Input: part model. Units: mm. Frame: model coordinates. Face numbers are marked on the shaded views. A direction names the side the tool comes from. Round coordinates to 2 decimals unless told otherwise and drop trailing zeros. Order: outer loops, then holes, each group sorted by start corner. A loop starts at its lowest first (then second) coordinate and runs counter-clockwise, first axis right, second up. Notation, with made-up numbers: (49, 88) -> (88, 88) arc R28 ccw to (88, 112) -> close; hole circle Ø3 at (-39, -21). An arc over 180 degrees is marked (long way). Use a Markdown table: item, result.
from build123d import *

# Parameters (mm, degrees)
F1_DEPTH      = 70
F3_DEPTH      = 40
F4_SIZE       = 1
F6_DEPTH      = 25
F6_DEPTH_BACK = 100
F7_R          = 4
F8_DEPTH      = 30
F8_DEPTH_BACK = 25
F10_R         = 5
F11_DEPTH     = 30
F11_TAPER     = 1
F13_START     = 25
F12_R         = 21.0146982342
F13_DEPTH     = 15


with BuildPart() as f1:
    # F0 (on Top) → F1 (new body)
    with BuildSketch(Plane.XY):
        Polygon((0, -15), (0, 0), (0, 15), (-10, 9.2264973081), (-10, -9.2264973081), align=None)
    extrude(amount=F1_DEPTH)

    # F2 (on Right) → F3 (join)
    with BuildSketch(Plane.YZ):
        with BuildLine():
            ThreePointArc((7, 35), (-4.9497474683, 39.9497474683), (0, 28))
            ThreePointArc((0, 28), (4.9497474683, 30.0502525317), (7, 35))
        make_face()
        with BuildLine():
            ThreePointArc((4, 35), (2.8284271247, 32.1715728753), (0, 31))
            ThreePointArc((0, 31), (-2.8284271247, 37.8284271247), (4, 35))
        make_face(mode=Mode.SUBTRACT)
        with BuildLine():
            ThreePointArc((4, 35), (-2.8284271247, 37.8284271247), (0, 31))
            ThreePointArc((0, 31), (2.8284271247, 32.1715728753), (4, 35))
        make_face()
    extrude(amount=F3_DEPTH)

    # F4
    f4_edges = [f1.edges().sort_by_distance(p)[0] for p in [
        (40, -7, 35),
    ]]
    chamfer(f4_edges, length=F4_SIZE)

    # F5 (on Top) → F6 (cut, two sides)
    with BuildSketch(Plane.XY) as f6_sk:
        Polygon((26, -4), (34, -4), (34, 4), (26, 4), (26, 0), align=None)
    extrude(amount=-F6_DEPTH, mode=Mode.SUBTRACT)
    extrude(f6_sk.sketch, amount=F6_DEPTH_BACK, mode=Mode.SUBTRACT)

    # F7 (on Right) → F8 (cut, two sides)
    with BuildSketch(Plane.YZ) as f8_sk:
        with Locations((0, 35)):
            Circle(F7_R)
    extrude(amount=F8_DEPTH, mode=Mode.SUBTRACT)
    extrude(f8_sk.sketch, amount=-F8_DEPTH_BACK, mode=Mode.SUBTRACT)

    # F10 (on offset) → F11 (join)
    with BuildSketch(Plane.XY.offset(70)):
        with Locations((-5, 0)):
            Circle(F10_R)
    extrude(amount=F11_DEPTH, taper=F11_TAPER)

    # F12 (on offset) → F13 (cut)
    with BuildSketch(Plane.XY.offset(70).offset(F13_START)):
        with Locations((-5, 0)):
            Circle(F12_R)
        Polygon((-2, -3), (-8, -3), (-8, 3), (-2, 3), (-2, 0), align=None, mode=Mode.SUBTRACT)
    extrude(amount=F13_DEPTH, mode=Mode.SUBTRACT)


solid = f1.part
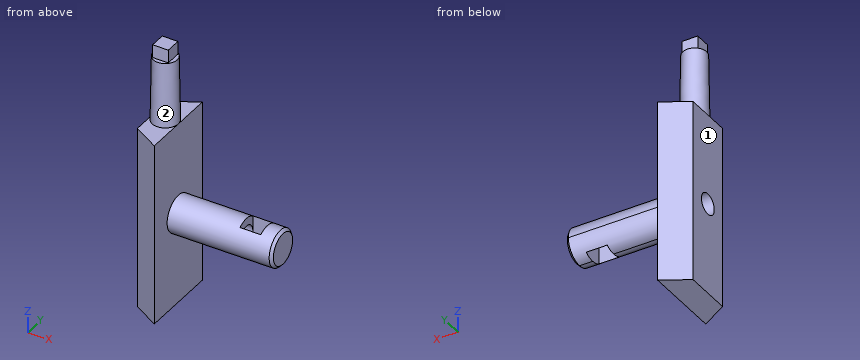
1) Line query: L1, parallel to Z at x = -0.5, y = 0; L2, parallel to Y at x = 15.5, z = 35; L3, parallel to X at y = 1, z = 16.5. Output: solid intervals per line, ascending. Write a range as [from, to].
Results found:
| item | result |
|---|---|
| L1 | z = [0, 31], [39, 95] |
| L2 | y = [-7, -4], [4, 7] |
| L3 | x = [-10, 0] |
2) Cut plane A-A on x = 25. Return loops of the section in (y, z), and give its area (3 significant figures).
Results found:
| item | result |
|---|---|
| outline | circle Ø14 at (0, 35); hole circle Ø8 at (0, 35) |
| area | 104 mm² |
3) Set-up query: the marked faces 1 and 2. Return all of +Z, -Z, +X, -X, +Y, -Y with unobstructed straight access to the full face (end or side cutting, diameter ignored); none if empty.
Results found:
| item | result |
|---|---|
| face 1 | +Z, -Z, -X, +Y, -Y |
| face 2 | +Z |
4) Cut plane B-B on y = 1.75. Count the separate pieces of the cut face and the enclosed holes in it, and give its area (3 significant figures).
Results found:
| item | result |
|---|---|
| separate pieces | 3 |
| enclosed holes | 0 |
| area | 1,130 mm² |
5) Pin query (flat end, axial travel): pin 1 Ø6.5 at (x, z) = (28.5, 33) entering from -Y; pin 2 Ø4 at (y, z) = (1, 96.5) entering from -X; pin 3 Ø5 at (y, z) = (11, 55.5) entering from +X. Return the tip coordinate at first contact, or that it passes through.
Results found:
| item | result |
|---|---|
| pin 1 | stops at y = -7 |
| pin 2 | stops at x = -9.57 |
| pin 3 | stops at x = 0 |
6) Cut plane C-C on x = 35. Return loops of the section in (y, z), and give its area (3 significant figures).
Results found:
| item | result |
|---|---|
| outline | circle Ø14 at (0, 35) |
| area | 154 mm² |
7) Cut plane D-D on y = -11.25. Return loops of the section in (x, z).
Results found:
| item | result |
|---|---|
| outline | (-6.5, 0) -> (0, 0) -> (0, 70) -> (-6.5, 70) -> close |
